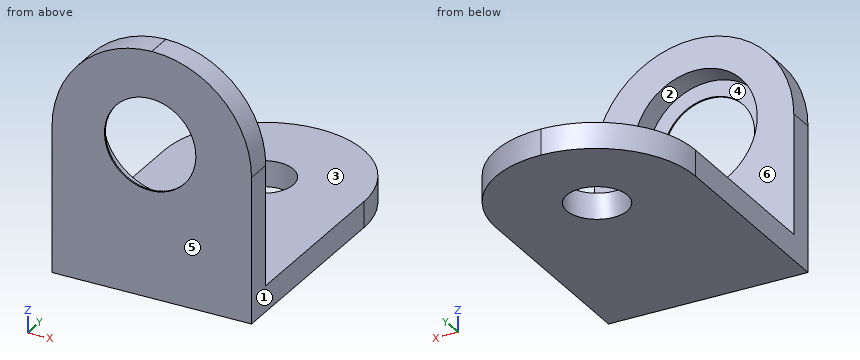
```python
from build123d import *

# Parameters (mm, degrees)
SKETCH2_R           = 2.5
BOSS_EXTRUDE1_DEPTH = 1.7
SKETCH3_W           = 13.1
SKETCH3_H           = 1.7
BOSS_EXTRUDE2_DEPTH = 18.3
SKETCH4_R           = 2
CUT_EXTRUDE1_DEPTH  = 18.3
FILLET1_R           = 6.545
SKETCH5_R           = 4.05
CUT_EXTRUDE2_DEPTH  = 1.6
SKETCH7_R           = 2.5
SKETCH7_R_2         = 1.5
BOSS_EXTRUDE4_DEPTH = 0.1
SKETCH9_R           = 3
SKETCH9_R_2         = 1.5
CUT_EXTRUDE3_DEPTH  = 2


with BuildPart() as part:
    # Sketch2 → Boss-Extrude1 (new body)
    with BuildSketch(Plane(origin=(0, 0, 0), x_dir=(1, 0, 0), z_dir=(0, 1, 0))):
        with BuildLine():
            Line((-6.446031746, 10), (6.653968254, 10))
            Line((6.653968254, 10), (6.653968254, 0.445))
            ThreePointArc((6.653968254, 0.445), (4.736982137, -4.183013883), (0.108968254, -6.1))
            Line((0.108968254, -6.1), (0.098968254, -6.1))
            ThreePointArc((0.098968254, -6.1), (-4.529045629, -4.183013883), (-6.446031746, 0.445))
            Line((-6.446031746, 0.445), (-6.446031746, 10))
        make_face()
        with Locations(Location((0, 0, 0), (0, 0, 270))):
            Circle(SKETCH2_R, mode=Mode.SUBTRACT)
    extrude(amount=BOSS_EXTRUDE1_DEPTH)

    # Sketch3 → Boss-Extrude2 (add)
    with BuildSketch(Plane(origin=(0, 1.7, 0), x_dir=(1, 0, 0), z_dir=(0, 1, 0))):
        with Locations((0.103968254, 9.15)):
            Rectangle(SKETCH3_W, SKETCH3_H)
    extrude(amount=BOSS_EXTRUDE2_DEPTH)

    # Sketch4 → Cut-Extrude1 (cut)
    with BuildSketch(Plane.XY.offset(-8.3)):
        with Locations((0.103968254, 13.3)):
            Circle(SKETCH4_R)
    extrude(amount=-CUT_EXTRUDE1_DEPTH, mode=Mode.SUBTRACT)

    # Fillet1
    fillet1_edges = [part.edges().sort_by_distance(p)[0] for p in [
        (-6.446031746, 20, -9.15),
        (6.653968254, 20, -9.15),
    ]]
    fillet(fillet1_edges, radius=FILLET1_R)

    # Sketch5 → Cut-Extrude2 (cut)
    with BuildSketch(Plane(origin=(0, 1.7, 0), x_dir=(1, 0, 0), z_dir=(0, 1, 0))):
        with Locations(Location((0, 0, 0), (0, 0, 270))):
            Circle(SKETCH5_R)
    extrude(amount=-CUT_EXTRUDE2_DEPTH, mode=Mode.SUBTRACT)

    # Sketch7 → Boss-Extrude4 (add)
    with BuildSketch(Plane.XZ):
        Circle(SKETCH7_R)
        with Locations(Location((0, 0, 0), (0, 0, 270))):
            Circle(SKETCH7_R_2, mode=Mode.SUBTRACT)
    extrude(amount=-BOSS_EXTRUDE4_DEPTH)

    # Sketch9 → Cut-Extrude3 (cut)
    with BuildSketch(Plane.XZ):
        with Locations(Location((0, 0, 0), (0, 0, 270))):
            Circle(SKETCH9_R)
        Circle(SKETCH9_R_2, mode=Mode.SUBTRACT)
    extrude(amount=-CUT_EXTRUDE3_DEPTH, mode=Mode.SUBTRACT)


solid = part.part
```
Build history of the part. All positions in model axes, mm. Face numbers are marked on the shaded views. A direction names the side the tool comes from. Round coordinates to 2 decimals unless told otherwise and drop trailing zeros. Order: outer loops, then holes, each group sorted by start corner. A loop starts at its lowest first (then second) coordinate and runs counter-clockwise, first axis right, second up. Notation, with made-up numbers: (-22.5, -3) -> (10.5, -3) arc R13 cw to (10.5, 20) -> close; hole circle Ø8 at (14.25, 49.5). An arc over 180 degrees is marked (long way). Answer in a Markdown table with one row per item.
1) Band-saw the part on B-B on x = -1.5. Give the cut face in (y, z), and give its area (3 significant figures).
Values:
| item | result |
|---|---|
| outline | (0, -10) -> (12.11, -10) -> (12.11, -8.3) -> (1.7, -8.3) -> (1.7, -3.76) -> (0.1, -3.76) -> (0.1, -2.6) -> (0, -2.6) -> close; (0, 2.6) -> (0.1, 2.6) -> (0.1, 3.76) -> (1.7, 3.76) -> (1.7, 5.9) -> (0, 5.9) -> close; (14.49, -10) -> (19.8, -10) -> (19.8, -8.3) -> (14.49, -8.3) -> close |
| area | 41.2 mm2 |
2) Wall check: L1, parallel to Z at x = -0.5, y = 4.5; L2, parallel to X at y = 1, z = 0; L3, parallel to Y at x = -4.25, z = 0.5. Give the ranges that are in metal, low to high.
Values:
| item | result |
|---|---|
| L1 | -10 to -8.3 |
| L2 | -6.43 to -4.05, 4.05 to 6.64 |
| L3 | 0 to 1.7 |
3) Mould opens along Z. For the marked faces 1, 2, 3 and 4 say: released by +Z, released by -Z, zero draft, split by the parting line, or undercut.
Values:
| item | result |
|---|---|
| face 1 | zero draft |
| face 2 | undercut |
| face 3 | released by +Z |
| face 4 | undercut |
4) Band-saw the part on D-D on z = 0. Give the cut face in (x, y), and give its area (3 significant figures).
Values:
| item | result |
|---|---|
| outline | (-6.43, 0) -> (-3, 0) -> (-3, 0.1) -> (-4.05, 0.1) -> (-4.05, 1.7) -> (-6.43, 1.7) -> close; (3, 0) -> (6.64, 0) -> (6.64, 1.7) -> (4.05, 1.7) -> (4.05, 0.1) -> (3, 0.1) -> close |
| area | 8.66 mm2 |
5) Which spindle directions (+Z, -Z, +X, -X, +Y, -Y) get a long thin tool onto all of the face, cutting with end or side? Do the marked faces 5 and 6. Say none if no direction does.
Values:
| item | result |
|---|---|
| face 5 | +Z, -Z, +X, -X, -Y |
| face 6 | +Z, +X, -X, +Y |
6) Band-saw the part on C-C on y = 5. Give the cut face in (x, z), and give its area (3 significant figures).
Values:
| item | result |
|---|---|
| outline | (-6.45, -10) -> (6.65, -10) -> (6.65, -8.3) -> (-6.45, -8.3) -> close |
| area | 22.3 mm2 |
7) Band-saw the part on A-A on z = 2.25. Give the cut face in (x, y), and give its area (3 significant figures).
Values:
| item | result |
|---|---|
| outline | (-5.87, 0) -> (-1.98, 0) -> (-1.98, 0.1) -> (-3.37, 0.1) -> (-3.37, 1.7) -> (-5.87, 1.7) -> close; (1.98, 0) -> (6.07, 0) -> (6.07, 1.7) -> (3.37, 1.7) -> (3.37, 0.1) -> (1.98, 0.1) -> close |
| area | 9.12 mm2 |
8) Pin check, flat tips, straight feed: P1, Ø6.5, axis at x = 0.5, z = 1.5, coming from the +Y side; P2, Ø4.5, axis at x = 0.1, y = 13.3, coming from the +Z side; P3, Ø5, axis at x = 0, z = 0, coming from the -Y side. Stop position of each tip, or through.
Values:
| item | result |
|---|---|
| P1 | y = 1.7 |
| P2 | z = -8.3 |
| P3 | through |
